Verification items for the finished model (mm, model axes). Face numbers are marked on the shaded views. A direction names the side the tool comes from. Round coordinates to 2 decimals unless told otherwise and drop trailing zeros. Order: outer loops, then holes, each group sorted by start corner. A loop starts at its lowest first (then second) coordinate and runs counter-clockwise, first axis right, second up. Notation, with made-up numbers: (83, 39.25) -> (101, 39.25) arc R31 ccw to (101, 68.25) -> close; hole circle Ø1 at (-36, 61). An arc over 180 degrees is marked (long way). Put each result on its own line as item: value.
from build123d import *

# Parameters (mm, degrees)
F0_R     = 12.7
F1_DEPTH = 12.7
F2_R     = 11.1125
F3_DEPTH = 63.5
F4_R     = 11.1125
F5_DEPTH = 10.16
F5_TAPER = 45


with BuildPart() as f1:
    # F0 (on Top) → F1 (new body)
    with BuildSketch(Plane.XY):
        Circle(F0_R)
    extrude(amount=-F1_DEPTH)

    # F2 (on face) → F3 (join)
    with BuildSketch(Plane(origin=(0, 0, -12.7), x_dir=(1, 0, 0), z_dir=(0, 0, -1))):
        Circle(F2_R)
    extrude(amount=F3_DEPTH)

    # F4 (on face) → F5 (join)
    with BuildSketch(Plane(origin=(0, 0, -76.2), x_dir=(1, 0, 0), z_dir=(0, 0, -1))):
        Circle(F4_R)
    extrude(amount=F5_DEPTH, taper=F5_TAPER)


solid = f1.part
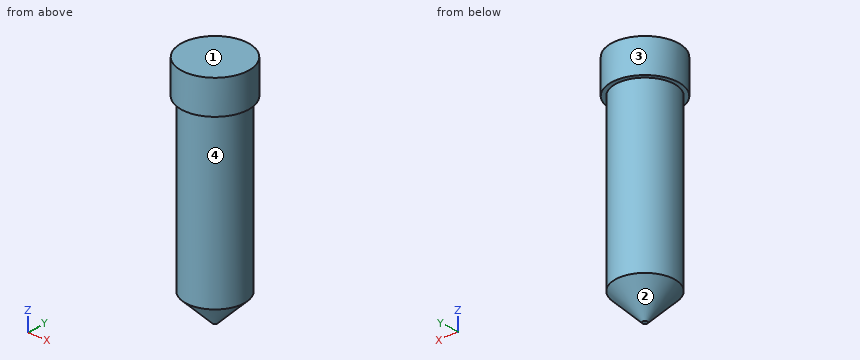
Item 1: Release check for a two-part mould opening along Y. For the marked faces 1 and 2 record: +Y half, -Y half, draft (parallel to the pull), parting line (faces both ways), or undercut.
Check sheet entries:
face 1: draft
face 2: parting line
Item 2: Tool access check on the marked faces 3 and 4. Record the directions out of +Z, -Z, +X, -X, +Y, -Y that give a thin tool (end or side, any length) a straight path to the whole face; none if there is none.
Check sheet entries:
face 3: +Z, -Z
face 4: -Z
Item 3: Gauge pin test, flat ends, axial feed: pin 1 Ø7.5 at (x, y) = (1.5, 5.5) entering from -Z; pin 2 Ø3 at (x, z) = (3, -41) entering from -Y; pin 3 Ø12 at (x, y) = (6, -7) entering from -Z. Record the tip position at first contact, or that the pin passes through.
Check sheet entries:
pin 1: stops at z = -85.36
pin 2: stops at y = -11.01
pin 3: stops at z = -84.09
Item 4: Section check A-A on x = 0. Record the boundary of the cut face in (y, z), then the cut area to 3 significant figures.
Check sheet entries:
outline: (-12.7, -12.7) -> (-11.11, -12.7) -> (-11.11, -76.2) -> (-0.95, -86.36) -> (0.95, -86.36) -> (11.11, -76.2) -> (11.11, -12.7) -> (12.7, -12.7) -> (12.7, 0) -> (-12.7, 0) -> close
area: 1,860 mm^2
Item 5: Section check B-B on z = -53. Record the boundary of the cut face in (x, y) (1 decimal), then the cut area to 3 significant figures.
Check sheet entries:
outline: circle Ø22.2 at (0, 0)
area: 388 mm^2
Item 6: Material ranges on L1, parallel to Z at x = 8, y = -9; L2, parallel to X at y = 1, z = -48; L3, parallel to X at y = 4.75, z = -80.5, recorded low to high. Write a range as [from, to].
Check sheet entries:
L1: z = [-12.7, 0]
L2: x = [-11.07, 11.07]
L3: x = [-4.88, 4.88]
